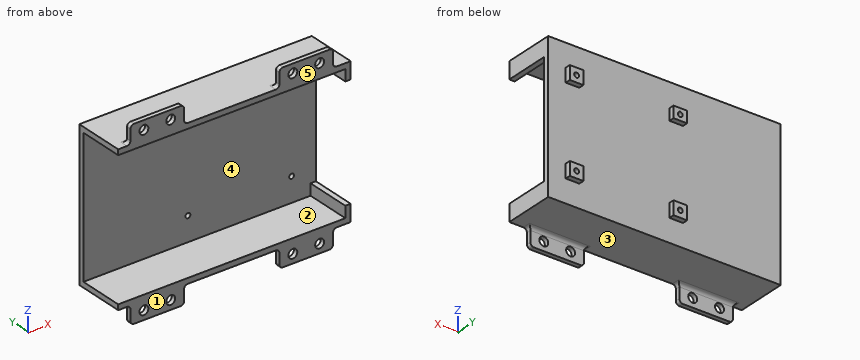
from build123d import *

# Parameters (mm, degrees)
SKETCH1_R                        = 2.54
SKETCH1_R_2                      = 6.35
MAINBASEPLATE_DEPTH              = 3
PIBATTERYBOXBOSS_EXTRUDE3_DEPTH  = 25.4
SKETCH7_W                        = 130
SKETCH7_H                        = 82.2
PIBATTERYTOPBOSS_EXTRUDE4_DEPTH  = 3
SKETCH8_W                        = 63.5
SKETCH8_H                        = 25.4
PIBATTERYWIRESCUT_EXTRUDE2_DEPTH = 13.16
SKETCH9_W                        = 7.62
SKETCH9_H                        = 7.62
SKETCH9_R                        = 1.35
SKETCH9_H_2                      = 6.437586206
PIBOARDBOSS_EXTRUDE5_DEPTH       = 3
SKETCH32_W                       = 712.395528774
SKETCH32_H                       = 524.196017535
CUT_EXTRUDE11_DEPTH              = 3
SKETCH33_W                       = 30
SKETCH33_H                       = 10
SKETCH33_R                       = 2.5
BOSS_EXTRUDE9_DEPTH              = 2.5
FILLET2_R                        = 2
CUT_EXTRUDE12_START              = -5
SKETCH9_2_R                      = 1.35
CUT_EXTRUDE12_DEPTH              = 5


with BuildPart() as part:
    # Sketch1 → mainbaseplate (new body)
    with BuildSketch(Plane(origin=(0, 0, 0), x_dir=(1, 0, 0), z_dir=(0, 1, 0))):
        with BuildLine():
            Line((-223.52, -111.125), (223.52, -111.125))
            ThreePointArc((223.52, -111.125), (227.112102448, -109.637102448), (228.6, -106.045))
            Line((228.6, -106.045), (228.6, 106.045))
            ThreePointArc((228.6, 106.045), (227.112102448, 109.637102448), (223.52, 111.125))
            Line((223.52, 111.125), (-223.52, 111.125))
            ThreePointArc((-223.52, 111.125), (-227.112102448, 109.637102448), (-228.6, 106.045))
            Line((-228.6, 106.045), (-228.6, -106.045))
            ThreePointArc((-228.6, -106.045), (-227.112102448, -109.637102448), (-223.52, -111.125))
        make_face()
        with Locations(Location((127, 36.5125, 0), (0, 0, 270))):
            Circle(SKETCH1_R, mode=Mode.SUBTRACT)
        with Locations(Location((127, -36.5125, 0), (0, 0, 270))):
            Circle(SKETCH1_R, mode=Mode.SUBTRACT)
        with Locations(Location((-142.24, 36.5125, 0), (0, 0, 270))):
            Circle(SKETCH1_R, mode=Mode.SUBTRACT)
        with Locations(Location((-142.24, -36.5125, 0), (0, 0, 270))):
            Circle(SKETCH1_R, mode=Mode.SUBTRACT)
        with Locations(Location((209.55, 0, 0), (0, 0, 270))):
            Circle(SKETCH1_R_2, mode=Mode.SUBTRACT)
    extrude(amount=MAINBASEPLATE_DEPTH)

    # Sketch6 → PiBatteryBoxBoss-Extrude3 (add)
    with BuildSketch(Plane(origin=(0, 3, 0), x_dir=(1, 0, 0), z_dir=(0, 1, 0))):
        Polygon((-63.5, -41.1), (66.5, -41.1), (66.5, 41.1), (-63.5, 41.1), (-63.5, 38.1), (63.5, 38.1), (63.5, -38.1), (-63.5, -38.1), align=None)
    extrude(amount=PIBATTERYBOXBOSS_EXTRUDE3_DEPTH)

    # Sketch7 → PibatterytopBoss-Extrude4 (add)
    with BuildSketch(Plane(origin=(0, 28.4, 0), x_dir=(1, 0, 0), z_dir=(0, 1, 0))):
        with Locations((1.5, 0)):
            Rectangle(SKETCH7_W, SKETCH7_H)
    extrude(amount=PIBATTERYTOPBOSS_EXTRUDE4_DEPTH)

    # Sketch8 → pibatterywiresCut-Extrude2 (cut)
    with BuildSketch(Plane(origin=(66.5, 0, 0), x_dir=(0, 0, -1), z_dir=(1, 0, 0))):
        with Locations((0, 15.7)):
            Rectangle(SKETCH8_W, SKETCH8_H)
    extrude(amount=-PIBATTERYWIRESCUT_EXTRUDE2_DEPTH, mode=Mode.SUBTRACT)

    # Sketch9 → PiBoardBoss-Extrude5 (add)
    # profile 1 of 4: a face of its own
    with BuildSketch(Plane(origin=(0, 31.4, 0), x_dir=(1, 0, 0), z_dir=(0, 1, 0))):
        with Locations((52.92, 24.511)):
            Rectangle(SKETCH9_W, SKETCH9_H)
        with Locations(Location((52.92, 24.511, 0), (0, 0, 270))):
            Circle(SKETCH9_R, mode=Mode.SUBTRACT)
    # profile 2 of 4: a face of its own
    with BuildSketch(Plane(origin=(0, 31.4, 0), x_dir=(1, 0, 0), z_dir=(0, 1, 0))):
        with Locations((52.92, -24.489)):
            Rectangle(SKETCH9_W, SKETCH9_H)
        with Locations(Location((52.92, -24.489, 0), (0, 0, 270))):
            Circle(SKETCH9_R, mode=Mode.SUBTRACT)
    # profile 3 of 4: a face of its own
    with BuildSketch(Plane(origin=(0, 31.4, 0), x_dir=(1, 0, 0), z_dir=(0, 1, 0))):
        with Locations((-5.08, 24.511)):
            Rectangle(SKETCH9_W, SKETCH9_H)
        with Locations(Location((-5.08, 24.511, 0), (0, 0, 270))):
            Circle(SKETCH9_R, mode=Mode.SUBTRACT)
    # profile 4 of 4: a face of its own
    with BuildSketch(Plane(origin=(0, 31.4, 0), x_dir=(1, 0, 0), z_dir=(0, 1, 0))):
        with Locations((-5.08, -24.489)):
            Rectangle(SKETCH9_W, SKETCH9_H_2)
        with Locations(Location((-5.08, -24.489, 0), (0, 0, 270))):
            Circle(SKETCH9_R, mode=Mode.SUBTRACT)
    extrude(amount=PIBOARDBOSS_EXTRUDE5_DEPTH)

    # Sketch32 → Cut-Extrude11 (cut)
    with BuildSketch(Plane.XZ):
        with Locations((-5.907824988, 36.768742763)):
            Rectangle(SKETCH32_W, SKETCH32_H)
    extrude(amount=-CUT_EXTRUDE11_DEPTH, mode=Mode.SUBTRACT)

    # Sketch33 → Boss-Extrude9 (add)
    # profile 1 of 4: a face of its own
    with BuildSketch(Plane.XZ.offset(-3)):
        with Locations((-41.638953423, 46.1)):
            Rectangle(SKETCH33_W, SKETCH33_H)
        with Locations(Location((-49.138953423, 46.1, 0), (0, 0, 270))):
            Circle(SKETCH33_R, mode=Mode.SUBTRACT)
        with Locations(Location((-34.138953423, 46.1, 0), (0, 0, 90))):
            Circle(SKETCH33_R, mode=Mode.SUBTRACT)
    # profile 2 of 4: a face of its own
    with BuildSketch(Plane.XZ.offset(-3)):
        with Locations((41.638953423, 46.1)):
            Rectangle(SKETCH33_W, SKETCH33_H)
        with Locations(Location((34.138953423, 46.1, 0), (0, 0, 270))):
            Circle(SKETCH33_R, mode=Mode.SUBTRACT)
        with Locations(Location((49.138953423, 46.1, 0), (0, 0, 90))):
            Circle(SKETCH33_R, mode=Mode.SUBTRACT)
    # profile 3 of 4: a face of its own
    with BuildSketch(Plane.XZ.offset(-3)):
        with Locations((41.638953423, -46.1)):
            Rectangle(SKETCH33_W, SKETCH33_H)
        with Locations(Location((49.138953423, -46.1, 0), (0, 0, 270))):
            Circle(SKETCH33_R, mode=Mode.SUBTRACT)
        with Locations(Location((34.138953423, -46.1, 0), (0, 0, 90))):
            Circle(SKETCH33_R, mode=Mode.SUBTRACT)
    # profile 4 of 4: a face of its own
    with BuildSketch(Plane.XZ.offset(-3)):
        with Locations((-41.638953423, -46.1)):
            Rectangle(SKETCH33_W, SKETCH33_H)
        with Locations(Location((-49.138953423, -46.1, 0), (0, 0, 90))):
            Circle(SKETCH33_R, mode=Mode.SUBTRACT)
        with Locations(Location((-34.138953423, -46.1, 0), (0, 0, 270))):
            Circle(SKETCH33_R, mode=Mode.SUBTRACT)
    extrude(amount=-BOSS_EXTRUDE9_DEPTH)

    # Fillet2
    fillet2_edges = [part.edges().sort_by_distance(p)[0] for p in [
        (-56.638953423, 4.25, 41.1),
        (-56.638953423, 4.25, 51.1),
        (-26.638953423, 4.25, 51.1),
        (-41.638953423, 5.5, 41.1),
        (-26.638953423, 4.25, 41.1),
        (56.638953423, 4.25, 51.1),
        (41.638953423, 5.5, 41.1),
        (56.638953423, 4.25, 41.1),
        (26.638953423, 4.25, 41.1),
        (26.638953423, 4.25, 51.1),
        (41.638953423, 5.5, -41.1),
        (26.638953423, 4.25, -41.1),
        (56.638953423, 4.25, -41.1),
        (56.638953423, 4.25, -51.1),
        (26.638953423, 4.25, -51.1),
        (-56.638953423, 4.25, -51.1),
        (-41.638953423, 5.5, -41.1),
        (-56.638953423, 4.25, -41.1),
        (-26.638953423, 4.25, -41.1),
        (-26.638953423, 4.25, -51.1),
    ]]
    fillet(fillet2_edges, radius=FILLET2_R)

    # Sketch9<2> → Cut-Extrude12 (cut)
    with BuildSketch(Plane(origin=(0, 31.4, 0), x_dir=(1, 0, 0), z_dir=(0, 1, 0)).offset(CUT_EXTRUDE12_START)):
        with Locations(Location((52.92, -24.489, 0), (0, 0, 90))):
            Circle(SKETCH9_2_R)
        with Locations(Location((-5.08, -24.489, 0), (0, 0, 90))):
            Circle(SKETCH9_2_R)
        with Locations(Location((-5.08, 24.511, 0), (0, 0, 90))):
            Circle(SKETCH9_2_R)
        with Locations(Location((52.92, 24.511, 0), (0, 0, 90))):
            Circle(SKETCH9_2_R)
    extrude(amount=CUT_EXTRUDE12_DEPTH, mode=Mode.SUBTRACT)


solid = part.part
Model file for the job. Use its own axes, mm. Face numbers are marked on the shaded views. A direction names the side the tool comes from. Coordinates: 2 decimals unless noted, no trailing zeros. Write each loop counter-clockwise with the first axis right and the second up, starting at its lowest first coordinate (ties: lowest second). Pieces come first, ordered by that corner, then holes. Notation, with made-up numbers: (22, 56.5) - (44, 56.5) arc R26 cw to (44, 74.5) - close; hole circle Ø5 at (61.25, 69). An arc over 180 degrees is marked (long way). Write each question's results on one line, items separated by ' | '. Start each with the question number.
1) Cut at B-B (z = -46.1). Write the cut outline in (x, y).
2) Probe line 1 along X through (y, z) = (4, -46); line 2 along Z through (x, y) = (-32, 19.5); line 3 along Y through (x, z) = (-27, 4). List the from-to ranges inside material, lowest first. Write a range as from..to.
3) Cut at D-D (x = 39). Write the cut outline in (y, z), then the cut area to 3 significant figures.
4) Mould opens along Z. For the marked faces 3, 4 and 5 say: pulls with the +Z half, pulls with the -Z half, needs draft (parallel to the pull), parting line crosses it, or undercut.
5) Cut at C-C (x = -5.08). Write the cut outline in (y, z), then the cut area to 3 significant figures.
6) Flat gauge pins, fed straight in: P1, Ø3, axis at x = -49.14, z = -46.1, coming from the +Y side; P2, Ø4, axis at x = 45.5, z = -6.5, coming from the +Y side; P3, Ø3, axis at x = 13, y = 21.5, coming from the +Z side; P4, Ø3.5, axis at x = 52, y = 32.5, coming from the -Z side. Where does each tip first touch, or does it go through?
7) Cut at A-A (y = 9.5). Write the cut outline in (x, z).
8) 3-axis set-ups, long thin cutter, end or side, ignore diameter. For the marked faces 1 and 2: which of +Z, -Z, +X, -X, +Y, -Y reach the whole face in a straight line?
Returned:
1) outline: (-56.64, 3) - (-51.64, 3) - (-51.64, 5.5) - (-56.64, 5.5) - close; (-46.64, 3) - (-36.64, 3) - (-36.64, 5.5) - (-46.64, 5.5) - close; (-31.64, 3) - (-26.64, 3) - (-26.64, 5.5) - (-31.64, 5.5) - close; (26.64, 3) - (31.64, 3) - (31.64, 5.5) - (26.64, 5.5) - close; (36.64, 3) - (46.64, 3) - (46.64, 5.5) - (36.64, 5.5) - close; (51.64, 3) - (56.64, 3) - (56.64, 5.5) - (51.64, 5.5) - close
2) line 1: -56.64..-51.64, -46.64..-36.64, -31.64..-26.64, 26.64..31.64, 36.64..46.64, 51.64..56.64 | line 2: -41.1..-38.1, 38.1..41.1 | line 3: 28.4..31.4
3) outline: (3, -51.1) - (5.5, -51.1) - (5.5, -43.1) arc R2 cw to (7.5, -41.1) - (31.4, -41.1) - (31.4, 41.1) - (7.5, 41.1) arc R2 cw to (5.5, 43.1) - (5.5, 51.1) - (3, 51.1) - (3, 38.1) - (28.4, 38.1) - (28.4, -38.1) - (3, -38.1) - close | area: 451 mm^2
4) face 3: pulls with the -Z half | face 4: undercut | face 5: needs draft
5) outline: (3, -41.1) - (31.4, -41.1) - (31.4, -28.32) - (34.4, -28.32) - (34.4, -25.86) - (28.4, -25.86) - (28.4, -38.1) - (3, -38.1) - close; (3, 38.1) - (28.4, 38.1) - (28.4, 25.84) - (34.4, 25.84) - (34.4, 27.71) - (31.4, 27.71) - (31.4, 41.1) - (3, 41.1) - close; (28.4, -23.16) - (34.4, -23.16) - (34.4, -20.7) - (31.4, -20.7) - (31.4, 21.27) - (34.4, 21.27) - (34.4, 23.14) - (28.4, 23.14) - close | area: 409 mm^2
6) P1: through | P2: y = 31.4 | P3: z = 41.1 | P4: z = -41.1
7) outline: (-63.5, -41.1) - (66.5, -41.1) - (66.5, -31.75) - (63.5, -31.75) - (63.5, -38.1) - (-63.5, -38.1) - close; (-63.5, 38.1) - (63.5, 38.1) - (63.5, 31.75) - (66.5, 31.75) - (66.5, 41.1) - (-63.5, 41.1) - close
8) face 1: +Z, -Z, +X, -X, -Y | face 2: -X, -Y
